Input: part model. Units: mm. Frame: model coordinates. Face numbers are marked on the shaded views. A direction names the side the tool comes from. Round coordinates to 2 decimals unless told otherwise and drop trailing zeros. Order: outer loops, then holes, each group sorted by start corner. A loop starts at its lowest first (then second) coordinate and runs counter-clockwise, first axis right, second up. Notation, with made-up numbers: (3.25, -30.5) -> (32.25, -30.5) arc R24 ccw to (32.25, -15.5) -> close; hole circle Ø7 at (54, 88.25). An arc over 180 degrees is marked (long way). Use a Markdown table: item, result.
from build123d import *

# Parameters (mm, degrees)
F1_DEPTH  = 31.75
F3_DEPTH  = 107.951
F5_DEPTH  = 6.35
F7_DEPTH  = 38.1
F8_DEPTH  = 25.4
F9_R      = 7.999836
F10_DEPTH = 127


with BuildPart() as f1:
    # F0 (on Front) → F1 (new body, symmetric)
    with BuildSketch(Plane.XZ):
        Polygon((0, 76.2), (0, 0), (107.95, 0), (107.95, 22.225), (15.875, 22.225), (15.875, 76.2), align=None)
    extrude(amount=F1_DEPTH, both=True)

    # F2 (on face) → F3 (cut, through all)
    with BuildSketch(Plane.YZ.offset(107.95)):
        Polygon((-12.7, 0), (12.7, 0), (19.05, 9.525), (-19.05, 9.525), align=None)
    extrude(amount=-F3_DEPTH, mode=Mode.SUBTRACT)

    # F4 (on Front) → F5 (join, symmetric)
    with BuildSketch(Plane.XZ):
        Polygon((92.075, 22.225), (15.875, 66.219091), (15.875, 22.225), align=None)
    extrude(amount=F5_DEPTH, both=True)

    # F6 (on face) → F7 (cut, symmetric)
    with BuildSketch(Plane(origin=(0, 0, 0), x_dir=(0, -1, 0), z_dir=(-1, 0, 0))):
        Polygon((-31.75, 60.325), (-12.7, 76.2), (-31.75, 76.2), align=None)
        Polygon((31.75, 76.2), (12.7, 76.2), (31.75, 60.325), align=None)
    extrude(amount=F7_DEPTH, both=True, mode=Mode.SUBTRACT)

    # F6 (on face) → F8 (cut)
    with BuildSketch(Plane(origin=(0, 0, 0), x_dir=(0, -1, 0), z_dir=(-1, 0, 0))):
        Polygon((-31.75, 60.325), (-12.7, 76.2), (-31.75, 76.2), align=None)
        Polygon((31.75, 76.2), (12.7, 76.2), (31.75, 60.325), align=None)
    extrude(amount=-F8_DEPTH, mode=Mode.SUBTRACT)

    # F9 (on Front) → F10 (cut, symmetric)
    with BuildSketch(Plane.XZ):
        with Locations((15.979823, 22.425991)):
            Circle(F9_R)
    extrude(amount=F10_DEPTH, both=True, mode=Mode.SUBTRACT)


solid = f1.part
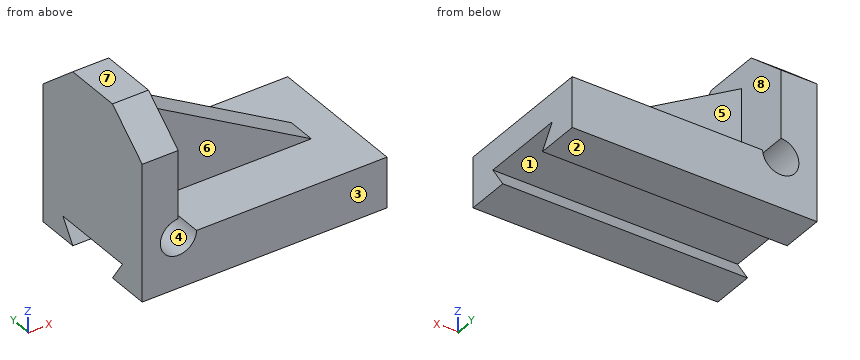
1) Draft query along Z for the marked faces 1, 2, 3 and 4. Return one class per face: released by +Z, released by -Z, zero draft, split by the parting line, or undercut.
Answer key:
| item | result |
|---|---|
| face 1 | undercut |
| face 2 | released by -Z |
| face 3 | zero draft |
| face 4 | undercut |
2) Cut plane A-A on x = 100. Return loops of the section in (y, z) (3 decimals).
Answer key:
| item | result |
|---|---|
| outline | (-31.75, 0) -> (-12.7, 0) -> (-19.05, 9.525) -> (19.05, 9.525) -> (12.7, 0) -> (31.75, 0) -> (31.75, 22.225) -> (-31.75, 22.225) -> close |
3) Cut plane C-C on z = 19. Return loops of the section in (x, y).
Answer key:
| item | result |
|---|---|
| outline | (0, -31.75) -> (8.75, -31.75) -> (8.75, 31.75) -> (0, 31.75) -> close; (23.21, -31.75) -> (107.95, -31.75) -> (107.95, 31.75) -> (23.21, 31.75) -> close |
4) Cut plane B-B on y = -10. Return loops of the section in (x, z) (3 decimals).
Answer key:
| item | result |
|---|---|
| outline | (0, 9.525) -> (107.95, 9.525) -> (107.95, 22.225) -> (23.977, 22.225) arc R8 cw (long way) to (15.875, 30.425) -> (15.875, 76.2) -> (0, 76.2) -> close |
5) Contact query for flat-ended pins moving along their axis: P1, Ø12, axis at x = 93, y = -23.5, coming from the +Z side (3 decimals); P2, Ø1, axis at x = 16.5, y = -25, coming from the +Z side; P3, Ø4, axis at x = 54.5, z = 32, coming from the -Y side. Output: stop coordinate, or through.
Answer key:
| item | result |
|---|---|
| P1 | stops at z = 22.225 |
| P2 | stops at z = 14.49 |
| P3 | stops at y = -6.35 |
6) Set-up query: the marked faces 5, 6, 7 and 8. Return all of +Z, -Z, +X, -X, +Y, -Y with unobstructed straight access to the full face (end or side cutting, diameter ignored); none if empty.
Answer key:
| item | result |
|---|---|
| face 5 | +Z, +X, +Y |
| face 6 | +Z, +X, -Y |
| face 7 | +Z, +X, -X, +Y, -Y |
| face 8 | +Z, +X |
7) Cut plane D-D on x = 17.5. Return loops of the section in (y, z) (3 decimals).
Answer key:
| item | result |
|---|---|
| outline | (-31.75, 0) -> (-12.7, 0) -> (-19.05, 9.525) -> (19.05, 9.525) -> (12.7, 0) -> (31.75, 0) -> (31.75, 14.572) -> (-31.75, 14.572) -> close; (-6.35, 30.28) -> (6.35, 30.28) -> (6.35, 65.281) -> (-6.35, 65.281) -> close |
8) Ray query, probe 1 along X at (y, z) = (2.5, 22); probe 2 along X at (y, z) = (-23.5, 63) (3 decimals); probe 3 along Z at (x, y) = (99.5, 20.5) (3 decimals). Return the intervals inside material, ascending.
Answer key:
| item | result |
|---|---|
| probe 1 | x = 0 to 7.99, 23.97 to 107.95 |
| probe 2 | x = 0 to 15.875 |
| probe 3 | z = 0 to 22.225 |
